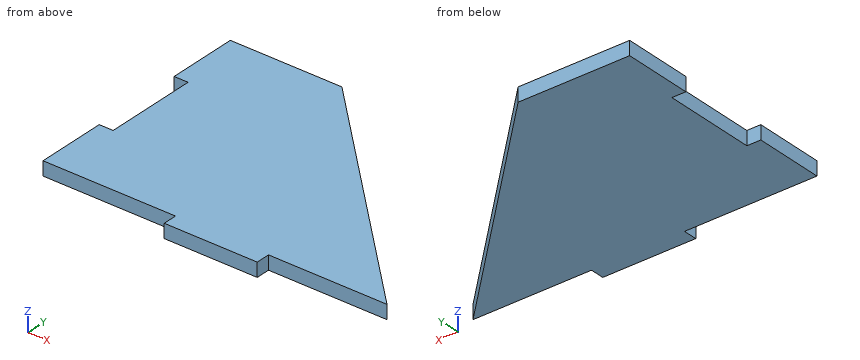
from build123d import *

# Parameters (mm, degrees)
SALIENTE_EXTRUIR1_DEPTH = 3
CROQUIS4_W              = 20
CROQUIS4_H              = 3
SALIENTE_EXTRUIR3_DEPTH = 3
CROQUIS5_W              = 3
CROQUIS5_H              = 20
CORTAR_EXTRUIR1_DEPTH   = 3


with BuildPart() as part:
    # Croquis1 → Saliente-Extruir1 (new body)
    with BuildSketch(Plane.XY):
        Polygon((35.5, -25), (-14.5, 25), (-38.5, 25), (-38.5, -25), align=None)
    extrude(amount=SALIENTE_EXTRUIR1_DEPTH)

    # Croquis4 → Saliente-Extruir3 (add)
    with BuildSketch(Plane.XY.offset(3)):
        with Locations((0, -26.5)):
            Rectangle(CROQUIS4_W, CROQUIS4_H)
    extrude(amount=-SALIENTE_EXTRUIR3_DEPTH)

    # Croquis5 → Cortar-Extruir1 (cut)
    with BuildSketch(Plane.XY.offset(3)):
        with Locations((-37, 0)):
            Rectangle(CROQUIS5_W, CROQUIS5_H)
    extrude(amount=-CORTAR_EXTRUIR1_DEPTH, mode=Mode.SUBTRACT)


solid = part.part
The listing builds one solid part. Answer for the finished solid, in the listing's coordinates (mm). Coordinates: 2 decimals unless noted, no trailing zeros. Loops run counter-clockwise (first coordinate to the right, second up) from the corner with the lowest first, then second, coordinate; pieces in that order, holes last. Notation, with made-up numbers: (55.5, 46) -> (87.5, 46) arc R20 cw to (87.5, 79) -> close; hole circle Ø7 at (-35.75, 87.5). An arc over 180 degrees is marked (long way). Answer in a Markdown table with one row per item. Add a question column.
1. The part is cut by section A-A, the plane z = 2.3. Write down the section's boundary in (x, y).
2. The part is cut by section C-C, the plane x = 22. Write down the section's boundary in (y, z).
3. Flat-ended cylindrical pins translate along their axes: P1, Ø0.9, axis at x = -20.5, z = 1, coming from the -Y side; P2, Ø1.5, axis at y = 1, z = 1.5, coming from the +X side; P3, Ø12, axis at x = 9, y = -22.5, coming from the -Z side. Find the tip coordinate at first contact, or state that the pin passes through.
4. The part is cut by section B-B, the plane y = 13. Write down the section's boundary in (x, z).
5. Consider line 1 (Y direction, x = -30.5, z = 2.3); line 2 (Y direction, x = -3, z = 0.35); line 3 (X direction, y = -19, z = 0.95). Determine where each line is inside the solid, lowest interval first. Write a range as [from, to].
Answer below:
| question | item | result |
|---|---|---|
| 1 | outline | (-38.5, -25) -> (-10, -25) -> (-10, -28) -> (10, -28) -> (10, -25) -> (35.5, -25) -> (-14.5, 25) -> (-38.5, 25) -> (-38.5, 10) -> (-35.5, 10) -> (-35.5, -10) -> (-38.5, -10) -> close |
| 2 | outline | (-25, 0) -> (-11.5, 0) -> (-11.5, 3) -> (-25, 3) -> close |
| 3 | P1 | y = -25 |
| 3 | P2 | x = 10.25 |
| 3 | P3 | z = 0 |
| 4 | outline | (-38.5, 0) -> (-2.5, 0) -> (-2.5, 3) -> (-38.5, 3) -> close |
| 5 | line 1 | [-25, 25] |
| 5 | line 2 | [-28, 13.5] |
| 5 | line 3 | [-38.5, 29.5] |
